Input: part model. Units: mm. Frame: model coordinates. Round coordinates to 2 decimals unless told otherwise and drop trailing zeros. Loops run counter-clockwise (first coordinate to the right, second up) from the corner with the lowest first, then second, coordinate; pieces in that order, holes last. Notation, with made-up numbers: (-10, 76.5) - (8, 76.5) arc R25 cw to (8, 89.5) - close; hole circle Ø9 at (-7, 8). An arc over 180 degrees is marked (long way). One line per question, with ' | ' between items. Start each with the question number.
Autodesk Inventor part; units mm, degrees
ref_plane "YZ Plane" through (0, 0, 0) normal (1, 0, 0) x (0, 1, 0)
ref_plane "XZ Plane" through (0, 0, 0) normal (0, 1, 0) x (-1, 0, 0)
ref_plane "XY Plane" through (0, 0, 0) normal (0, 0, 1) x (1, 0, 0)
sketch "Эскиз1" plane through (0, 0, 0) normal (0, 1, 0) x (-1, 0, 0)
  line L0 (21.1, -21.1) -> (-21.1, -21.1)
  line L1 (-21.1, -21.1) -> (-21.1, 21.1)
  line L2 (-21.1, 21.1) -> (21.1, 21.1)
  line L3 (21.1, 21.1) -> (21.1, -21.1)
  line L4 (21.1, -21.1) -> (-21.1, 21.1) construction
  line L5 (-21.1, -21.1) -> (21.1, 21.1) construction
  line L6 (-15.55, 15.55) -> (15.55, 15.55) construction
  line L7 (15.55, 15.55) -> (15.55, -15.55) construction
  line L8 (15.55, -15.55) -> (-15.55, -15.55) construction
  line L9 (-15.55, -15.55) -> (-15.55, 15.55) construction
  line L10 (-15.55, 15.55) -> (15.55, -15.55) construction
  line L11 (15.55, 15.55) -> (-15.55, -15.55) construction
  circle A0 centre (-15.55, -15.55) radius 1.5
  circle A1 centre (15.55, -15.55) radius 1.5
  circle A2 centre (15.55, 15.55) radius 1.5
  circle A3 centre (-15.55, 15.55) radius 1.5
  point P0 (0, 0)
  dimension "d0" = 42.2
  dimension "d1" = 42.2
  dimension "d2" = 31.1
  dimension "d3" = 31.1
  dimension "d4" = 3
  dimension "d5" = 3
  dimension "d6" = 3
  dimension "d7" = 3
extrude "Выдавливание1" add sketch "Эскиз1" along normal blind 32
chamfer "Фаска1" distance 4.5 angle 45 4 edges at (21.1, 16, -21.1) (21.1, 16, 21.1) (-21.1, 16, 21.1) (-21.1, 16, -21.1)
thread "Резьба1"
thread "Резьба2"
thread "Резьба3"
thread "Резьба4"
properties part number "Top"
(1) Line query: line 1 along Z through (x, y) = (15.55, 17); line 2 along Z through (x, y) = (15, 7). Output: solid intervals per line, ascending. Write a range as from..to.
(2) Section C-C, the plane y = 22. Output: boundary loops of the cut face in (x, z), plus the area to 3 significant figures.
(3) Pin query (flat end, axial travel): P1, Ø1.8, axis at x = 15.55, z = 15.55, coming from the -Y side. Return the tip coordinate at first contact, or that it passes through.
(4) Pull-direction query (Z, two-part tool) for faces 1 (the face through (-18.9, 15.8, 18.8)), 2 (the face through (21.1, 16, 0)), 3 (the face through (-16.2, 15.8, -14.2)); classes: released by +Z, released by -Z, zero draft, split by the parting line, or undercut.
(5) Section A-A, the plane x = 15.55. Output: boundary loops of the cut face in (y, z).
(6) Section B-B, the plane z = -15.55. Output: boundary loops of the cut face in (x, y), plus the area to 3 significant figures.
Derived:
1) line 1: z = -21.1..-17.05, -14.05..14.05, 17.05..21.1 | line 2: z = -21.1..-16.95, -14.15..14.15, 16.95..21.1
2) outline: (-21.1, -16.6) - (-16.6, -21.1) - (16.6, -21.1) - (21.1, -16.6) - (21.1, 16.6) - (16.6, 21.1) - (-16.6, 21.1) - (-21.1, 16.6) - close; hole circle Ø3 at (-15.55, -15.55); hole circle Ø3 at (-15.55, 15.55); hole circle Ø3 at (15.55, -15.55); hole circle Ø3 at (15.55, 15.55) | area: 1,710 mm²
3) P1: passes through
4) face 1: released by +Z | face 2: zero draft | face 3: undercut
5) outline: (0, -21.1) - (32, -21.1) - (32, -17.05) - (0, -17.05) - close; (0, -14.05) - (32, -14.05) - (32, 14.05) - (0, 14.05) - close; (0, 17.05) - (32, 17.05) - (32, 21.1) - (0, 21.1) - close
6) outline: (-21.1, 0) - (-17.05, 0) - (-17.05, 32) - (-21.1, 32) - close; (-14.05, 0) - (14.05, 0) - (14.05, 32) - (-14.05, 32) - close; (17.05, 0) - (21.1, 0) - (21.1, 32) - (17.05, 32) - close | area: 1,160 mm²
